The model under review builds one solid part; all positions refer to its coordinate system, in mm. Face numbers are marked on the shaded views. Round coordinates to 2 decimals unless told otherwise and drop trailing zeros. Write each loop counter-clockwise with the first axis right and the second up, starting at its lowest first coordinate (ties: lowest second). Pieces come first, ordered by that corner, then holes. Notation, with made-up numbers: (79.25, -33.5) - (116.25, -33.5) arc R21 cw to (116.25, -17.5) - close; hole circle Ø11 at (62, -29.75). An arc over 180 degrees is marked (long way). Return JSON: item names as keys, results as strings.
from build123d import *

# Parameters (mm, degrees)
F1_DEPTH = 7


with BuildPart() as f1:
    # F0 (on Top) → F1 (new body)
    with BuildSketch(Plane.XY):
        with BuildLine():
            ThreePointArc((9.6561832522, 5.575), (10.7700729631, 2.8858323529), (11.15, 0))
            ThreePointArc((11.15, 0), (10.7700729631, -2.8858323529), (9.6561832522, -5.575))
            ThreePointArc((9.6561832522, -5.575), (11.7583450993, -4.4386309052), (13.9764549062, -3.549581955))
            ThreePointArc((13.9764549062, -3.549581955), (14.308798821, -1.7886028346), (14.4201533903, 0))
            ThreePointArc((14.4201533903, 0), (14.3024193489, 1.8389194019), (13.9511397154, 3.6478109107))
            ThreePointArc((13.9511397154, 3.6478109107), (11.7522539794, 4.4968380812), (9.6561832522, 5.575))
        make_face()
        with BuildLine():
            ThreePointArc((10.0622555989, 10.3291740261), (9.7231396716, 7.9637101099), (9.6561832522, 5.575))
            ThreePointArc((9.6561832522, 5.575), (11.7522539794, 4.4968380812), (13.9511397154, 3.6478109107))
            ThreePointArc((13.9511397154, 3.6478109107), (12.4627822697, 7.2539562928), (10.0622555989, 10.3291740261))
        make_face()
        with BuildLine():
            ThreePointArc((0, 11.15), (5.575, 9.6561832522), (9.6561832522, 5.575))
            ThreePointArc((9.6561832522, 5.575), (9.7231396716, 7.9637101099), (10.0622555989, 10.3291740261))
            ThreePointArc((10.0622555989, 10.3291740261), (7.1661079009, 12.5135015624), (3.8164729409, 13.9059468606))
            ThreePointArc((3.8164729409, 13.9059468606), (1.9817509747, 12.4261695385), (0, 11.15))
        make_face()
        with BuildLine():
            ThreePointArc((10.1346667746, -10.25813595), (9.7705030047, -7.9293314573), (9.6561832522, -5.575))
            ThreePointArc((9.6561832522, -5.575), (5.575, -9.6561832522), (0, -11.15))
            ThreePointArc((0, -11.15), (2.0352054277, -12.4023410151), (3.9141993072, -13.8787559811))
            ThreePointArc((3.9141993072, -13.8787559811), (7.2539562928, -12.4627822697), (10.1346667746, -10.25813595))
        make_face()
        with BuildLine():
            ThreePointArc((13.9764549062, -3.549581955), (11.7583450993, -4.4386309052), (9.6561832522, -5.575))
            ThreePointArc((9.6561832522, -5.575), (9.7705030047, -7.9293314573), (10.1346667746, -10.25813595))
            ThreePointArc((10.1346667746, -10.25813595), (12.5135015624, -7.1661079009), (13.9764549062, -3.549581955))
        make_face()
        with BuildLine():
            ThreePointArc((-3.9141993072, 13.8787559811), (-2.0352054277, 12.4023410151), (0, 11.15))
            ThreePointArc((0, 11.15), (1.9817509747, 12.4261695385), (3.8164729409, 13.9059468606))
            ThreePointArc((3.8164729409, 13.9059468606), (-0.0507192927, 14.4200641938), (-3.9141993072, 13.8787559811))
        make_face()
        with BuildLine():
            ThreePointArc((-9.6561832522, 5.575), (-5.575, 9.6561832522), (0, 11.15))
            ThreePointArc((0, 11.15), (-2.0352054277, 12.4023410151), (-3.9141993072, 13.8787559811))
            ThreePointArc((-3.9141993072, 13.8787559811), (-7.2539562928, 12.4627822697), (-10.1346667746, 10.25813595))
            ThreePointArc((-10.1346667746, 10.25813595), (-9.7705030047, 7.9293314573), (-9.6561832522, 5.575))
        make_face()
        with BuildLine():
            ThreePointArc((10.0622555989, 10.3291740261), (12.4627822697, 7.2539562928), (13.9511397154, 3.6478109107))
            ThreePointArc((13.9511397154, 3.6478109107), (22.5646732179, 2.6278419368), (30.9082990141, 4.9979062145))
            ThreePointArc((30.9082990141, 4.9979062145), (16.7608876912, 8.7297196525), (18.4895315816, 23.2585691931))
            ThreePointArc((18.4895315816, 23.2585691931), (13.039109397, 17.5999976189), (10.0622555989, 10.3291740261))
        make_face()
        with BuildLine():
            ThreePointArc((-3.8164729409, -13.9059468606), (-1.9817509747, -12.4261695385), (0, -11.15))
            ThreePointArc((0, -11.15), (-5.575, -9.6561832522), (-9.6561832522, -5.575))
            ThreePointArc((-9.6561832522, -5.575), (-9.7231396716, -7.9637101099), (-10.0622555989, -10.3291740261))
            ThreePointArc((-10.0622555989, -10.3291740261), (-7.1661079009, -12.5135015624), (-3.8164729409, -13.9059468606))
        make_face()
        with BuildLine():
            ThreePointArc((3.9141993072, -13.8787559811), (2.0352054277, -12.4023410151), (0, -11.15))
            ThreePointArc((0, -11.15), (-1.9817509747, -12.4261695385), (-3.8164729409, -13.9059468606))
            ThreePointArc((-3.8164729409, -13.9059468606), (0.0507192927, -14.4200641938), (3.9141993072, -13.8787559811))
        make_face()
        with BuildLine():
            ThreePointArc((13.9764549062, -3.549581955), (12.5135015624, -7.1661079009), (10.1346667746, -10.25813595))
            ThreePointArc((10.1346667746, -10.25813595), (13.5581144833, -18.2276592665), (19.7824632545, -24.2684190267))
            ThreePointArc((19.7824632545, -24.2684190267), (15.9406028326, -10.1504947043), (29.3872775678, -4.3831194572))
            ThreePointArc((29.3872775678, -4.3831194572), (21.761599743, -2.4922011711), (13.9764549062, -3.549581955))
        make_face()
        with BuildLine():
            ThreePointArc((-13.9764549062, 3.549581955), (-11.7583450993, 4.4386309052), (-9.6561832522, 5.575))
            ThreePointArc((-9.6561832522, 5.575), (-9.7705030047, 7.9293314573), (-10.1346667746, 10.25813595))
            ThreePointArc((-10.1346667746, 10.25813595), (-12.5135015624, 7.1661079009), (-13.9764549062, 3.549581955))
        make_face()
        with BuildLine():
            ThreePointArc((-9.6561832522, -5.575), (-11.15, 0), (-9.6561832522, 5.575))
            ThreePointArc((-9.6561832522, 5.575), (-11.7583450993, 4.4386309052), (-13.9764549062, 3.549581955))
            ThreePointArc((-13.9764549062, 3.549581955), (-14.4200641938, -0.0507192927), (-13.9511397154, -3.6478109107))
            ThreePointArc((-13.9511397154, -3.6478109107), (-11.7522539794, -4.4968380812), (-9.6561832522, -5.575))
        make_face()
        with BuildLine():
            ThreePointArc((-3.9141993072, 13.8787559811), (-0.0507192927, 14.4200641938), (3.8164729409, 13.9059468606))
            ThreePointArc((3.8164729409, 13.9059468606), (9.0065587346, 20.8555012032), (11.1258357595, 29.2663252412))
            ThreePointArc((11.1258357595, 29.2663252412), (0.8202848586, 18.8802143568), (-10.8977459861, 27.6416886503))
            ThreePointArc((-10.8977459861, 27.6416886503), (-8.722490346, 20.0921987899), (-3.9141993072, 13.8787559811))
        make_face()
        with BuildLine():
            ThreePointArc((31.5557621135, 5.3438167478), (31.2334654211, 5.168175766), (30.9082990141, 4.9979062145))
            ThreePointArc((30.9082990141, 4.9979062145), (31.2348780107, 5.1655317307), (31.5557621135, 5.3438167478))
        make_face()
        with BuildLine():
            ThreePointArc((18.4895315816, 23.2585691931), (16.7608876912, 8.7297196525), (30.9082990141, 4.9979062145))
            ThreePointArc((30.9082990141, 4.9979062145), (31.2334654211, 5.168175766), (31.5557621135, 5.3438167478))
            ThreePointArc((31.5557621135, 5.3438167478), (35.6369453657, 9.425), (37.1307621135, 15))
            ThreePointArc((37.1307621135, 15), (30.497136742, 25.1943543305), (18.4895315816, 23.2585691931))
        make_face()
        with BuildLine():
            ThreePointArc((-10.0622555989, -10.3291740261), (-9.7231396716, -7.9637101099), (-9.6561832522, -5.575))
            ThreePointArc((-9.6561832522, -5.575), (-11.7522539794, -4.4968380812), (-13.9511397154, -3.6478109107))
            ThreePointArc((-13.9511397154, -3.6478109107), (-12.4627822697, -7.2539562928), (-10.0622555989, -10.3291740261))
        make_face()
        with BuildLine():
            ThreePointArc((3.9141993072, -13.8787559811), (0.0507192927, -14.4200641938), (-3.8164729409, -13.9059468606))
            ThreePointArc((-3.8164729409, -13.9059468606), (-9.0065587346, -20.8555012032), (-11.1258357595, -29.2663252412))
            ThreePointArc((-11.1258357595, -29.2663252412), (-0.8202848586, -18.8802143568), (10.8977459861, -27.6416886503))
            ThreePointArc((10.8977459861, -27.6416886503), (8.722490346, -20.0921987899), (3.9141993072, -13.8787559811))
        make_face()
        with BuildLine():
            ThreePointArc((20.4057621135, -24.6561832522), (20.0925042151, -24.4648866199), (19.7824632545, -24.2684190267))
            ThreePointArc((19.7824632545, -24.2684190267), (20.0909207082, -24.467431976), (20.4057621135, -24.6561832522))
        make_face()
        with BuildLine():
            ThreePointArc((29.3872775678, -4.3831194572), (15.9406028326, -10.1504947043), (19.7824632545, -24.2684190267))
            ThreePointArc((19.7824632545, -24.2684190267), (20.0925042151, -24.4648866199), (20.4057621135, -24.6561832522))
            ThreePointArc((20.4057621135, -24.6561832522), (31.5557621135, -24.6561832522), (37.1307621135, -15))
            ThreePointArc((37.1307621135, -15), (34.98923444, -8.4296174889), (29.3872775678, -4.3831194572))
        make_face()
        with BuildLine():
            ThreePointArc((-13.9764549062, 3.549581955), (-12.5135015624, 7.1661079009), (-10.1346667746, 10.25813595))
            ThreePointArc((-10.1346667746, 10.25813595), (-13.5581144833, 18.2276592665), (-19.7824632545, 24.2684190267))
            ThreePointArc((-19.7824632545, 24.2684190267), (-16.1462938443, 20.2541158972), (-14.8307621135, 15))
            ThreePointArc((-14.8307621135, 15), (-19.4103796024, 5.9915276735), (-29.3872775678, 4.3831194572))
            ThreePointArc((-29.3872775678, 4.3831194572), (-21.761599743, 2.4922011711), (-13.9764549062, 3.549581955))
        make_face()
        with BuildLine():
            ThreePointArc((11.15, 30), (11.140961206, 29.6330623859), (11.1258357595, 29.2663252412))
            ThreePointArc((11.1258357595, 29.2663252412), (11.1439573025, 29.6329637068), (11.15, 30))
        make_face()
        with BuildLine():
            ThreePointArc((-10.8977459861, 27.6416886503), (0.8202848586, 18.8802143568), (11.1258357595, 29.2663252412))
            ThreePointArc((11.1258357595, 29.2663252412), (11.140961206, 29.6330623859), (11.15, 30))
            ThreePointArc((11.15, 30), (-1.185882004, 41.0867571396), (-10.8977459861, 27.6416886503))
        make_face()
        with BuildLine():
            ThreePointArc((-10.0622555989, -10.3291740261), (-12.4627822697, -7.2539562928), (-13.9511397154, -3.6478109107))
            ThreePointArc((-13.9511397154, -3.6478109107), (-22.5646732179, -2.6278419368), (-30.9082990141, -4.9979062145))
            ThreePointArc((-30.9082990141, -4.9979062145), (-20.0909207082, -5.532568024), (-14.8307621135, -15))
            ThreePointArc((-14.8307621135, -15), (-15.7864077831, -19.5163746285), (-18.4895315816, -23.2585691931))
            ThreePointArc((-18.4895315816, -23.2585691931), (-13.039109397, -17.5999976189), (-10.0622555989, -10.3291740261))
        make_face()
        with BuildLine():
            ThreePointArc((-11.15, -30), (-11.140961206, -29.6330623859), (-11.1258357595, -29.2663252412))
            ThreePointArc((-11.1258357595, -29.2663252412), (-11.1439573025, -29.6329637068), (-11.15, -30))
        make_face()
        with BuildLine():
            ThreePointArc((10.8977459861, -27.6416886503), (-0.8202848586, -18.8802143568), (-11.1258357595, -29.2663252412))
            ThreePointArc((-11.1258357595, -29.2663252412), (-11.140961206, -29.6330623859), (-11.15, -30))
            ThreePointArc((-11.15, -30), (0, -41.15), (11.15, -30))
            ThreePointArc((11.15, -30), (11.0867571396, -28.814117996), (10.8977459861, -27.6416886503))
        make_face()
        with BuildLine():
            ThreePointArc((-20.4057621135, 24.6561832522), (-20.0925042151, 24.4648866199), (-19.7824632545, 24.2684190267))
            ThreePointArc((-19.7824632545, 24.2684190267), (-20.0909207082, 24.467431976), (-20.4057621135, 24.6561832522))
        make_face()
        with BuildLine():
            ThreePointArc((-14.8307621135, 15), (-16.1462938443, 20.2541158972), (-19.7824632545, 24.2684190267))
            ThreePointArc((-19.7824632545, 24.2684190267), (-20.0925042151, 24.4648866199), (-20.4057621135, 24.6561832522))
            ThreePointArc((-20.4057621135, 24.6561832522), (-36.175116444, 19.5163746285), (-29.3872775678, 4.3831194572))
            ThreePointArc((-29.3872775678, 4.3831194572), (-19.4103796024, 5.9915276735), (-14.8307621135, 15))
        make_face()
        with BuildLine():
            ThreePointArc((-31.5557621135, -5.3438167478), (-31.2334654211, -5.168175766), (-30.9082990141, -4.9979062145))
            ThreePointArc((-30.9082990141, -4.9979062145), (-31.2348780107, -5.1655317307), (-31.5557621135, -5.3438167478))
        make_face()
        with BuildLine():
            ThreePointArc((-14.8307621135, -15), (-20.0909207082, -5.532568024), (-30.9082990141, -4.9979062145))
            ThreePointArc((-30.9082990141, -4.9979062145), (-31.2334654211, -5.168175766), (-31.5557621135, -5.3438167478))
            ThreePointArc((-31.5557621135, -5.3438167478), (-34.98923444, -21.5703825111), (-18.4895315816, -23.2585691931))
            ThreePointArc((-18.4895315816, -23.2585691931), (-15.7864077831, -19.5163746285), (-14.8307621135, -15))
        make_face()
    extrude(amount=F1_DEPTH)


solid = f1.part
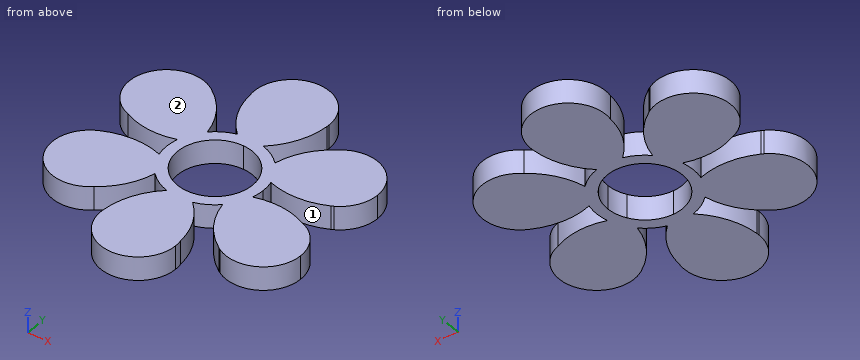
(1) Add section C-C (x = -6.5). Write out the cut boundary in (y, z).
Filled in:
{"outline": "(-39.06, 0) - (-16.79, 0) - (-16.79, 7) - (-39.06, 7) - close; (-12.87, 0) - (-9.06, 0) - (-9.06, 7) - (-12.87, 7) - close; (9.06, 0) - (12.87, 0) - (12.87, 7) - (9.06, 7) - close; (16.61, 0) - (39.06, 0) - (39.06, 7) - (16.61, 7) - close"}
(2) Wall thickness on line 1 (Y direction, x = -6, z = 6.75); line 2 (X direction, y = 11.5, z = 5); line 3 (Y direction, x = -9, z = 0.5): over which ranges is each line inside the solid? List them lowest first.
Filled in:
{"line 1": "y = -39.4 to -16.17, -13.11 to -9.4, 9.4 to 13.11, 16 to 39.4", "line 2": "x = -36.57 to -10.44, -8.7 to 8.7, 10.33 to 36.57", "line 3": "y = -36.58 to -20.84, -11.27 to -6.58, 6.58 to 11.27, 20.66 to 36.58"}
(3) Add section D-D (y = -31.5). Write out the cut boundary in (x, z), plus the area to 3 significant figures.
Filled in:
{"outline": "(-11.05, 0) - (11.05, 0) - (11.05, 7) - (-11.05, 7) - close", "area": "155 mm2"}
(4) Clearance check with flat-ended pins moving along their axes: pin 1 Ø1 at (x, z) = (-7.5, 3) entering from +Y; pin 2 Ø1 at (x, z) = (4, 3.5) entering from +Y; pin 3 Ø1.5 at (y, z) = (-24.5, 1.5) entering from +X. State where each tip first meets the part, or that it passes through.
Filled in:
{"pin 1": "stops at y = 38.68", "pin 2": "stops at y = 40.59", "pin 3": "stops at x = 32.89"}
(5) Add section A-A (x = 28). Write out the cut boundary in (y, z), plus the area to 3 significant figures.
Filled in:
{"outline": "(-25.97, 0) - (-3.8, 0) - (-3.8, 7) - (-25.97, 7) - close; (3.76, 0) - (25.97, 0) - (25.97, 7) - (3.76, 7) - close", "area": "311 mm2"}
(6) Add section B-B (y = -1.5). Write out the cut boundary in (x, z).
Filled in:
{"outline": "(-14.34, 0) - (-11.05, 0) - (-11.05, 7) - (-14.34, 7) - close; (11.05, 0) - (14.34, 0) - (14.34, 7) - (11.05, 7) - close"}
(7) Mouldability with a two-part tool opening along Y and no side actions: class the marked faces 1 and 2 as released by +Y, released by -Y, zero draft, split by the parting line, or undercut.
Filled in:
{"face 1": "undercut", "face 2": "zero draft"}
